Work out the finished part from the listing and answer in its coordinate system (mm). A direction names the side the tool comes from. Round coordinates to 2 decimals unless told otherwise and drop trailing zeros. Order: outer loops, then holes, each group sorted by start corner. A loop starts at its lowest first (then second) coordinate and runs counter-clockwise, first axis right, second up. Notation, with made-up numbers: M -7,-13.5 L 35,-13.5 A31 ccw 35,16.5 Z; hole C 86,85 d3. An arc over 180 degrees is marked long. Return JSON: item names as keys, results as strings.
from build123d import *

# Parameters (mm, degrees)
F0_W      = 205
F0_H      = 205
F0_W_2    = 195
F0_H_2    = 195
F1_DEPTH  = 200
F0_R      = 1.5
F0_W_3    = 55
F0_H_3    = 55
F2_DEPTH  = 3
F0_W_4    = 49
F0_H_4    = 49
F3_DEPTH  = 24
F4_W      = 46
F4_H      = 14
F5_DEPTH  = 60
F6_W      = 46
F6_H      = 14
F7_DEPTH  = 60
F8_W      = 49
F8_H      = 49
F9_DEPTH  = 4
F10_W     = 55
F10_H     = 55
F10_W_2   = 50
F10_H_2   = 50
F11_DEPTH = 150


with BuildPart() as f1:
    # F0 (on Top) → F1 (new body)
    with BuildSketch(Plane.XY):
        Rectangle(F0_W, F0_H)
        Rectangle(F0_W_2, F0_H_2, mode=Mode.SUBTRACT)
    extrude(amount=F1_DEPTH)

    # F0 (on Top) → F2 (join)
    with BuildSketch(Plane.XY):
        Rectangle(F0_W_2, F0_H_2)
        with Locations((-95.5, -95.5)):
            Circle(F0_R, mode=Mode.SUBTRACT)
        with Locations((-10, -48.9040691386)):
            Circle(F0_R, mode=Mode.SUBTRACT)
        with Locations((-48.9040691386, -10)):
            Circle(F0_R, mode=Mode.SUBTRACT)
        with Locations((95.5, -95.5)):
            Circle(F0_R, mode=Mode.SUBTRACT)
        with Locations((10, -48.9040691386)):
            Circle(F0_R, mode=Mode.SUBTRACT)
        with Locations((48.9040691386, -10)):
            Circle(F0_R, mode=Mode.SUBTRACT)
        with Locations((-48.9040691386, 10)):
            Circle(F0_R, mode=Mode.SUBTRACT)
        with Locations((-10, 48.9040691386)):
            Circle(F0_R, mode=Mode.SUBTRACT)
        with Locations((-95.5, 95.5)):
            Circle(F0_R, mode=Mode.SUBTRACT)
        Rectangle(F0_W_3, F0_H_3, mode=Mode.SUBTRACT)
        with Locations((48.9040691386, 10)):
            Circle(F0_R, mode=Mode.SUBTRACT)
        with Locations((10, 48.9040691386)):
            Circle(F0_R, mode=Mode.SUBTRACT)
        with Locations((95.5, 95.5)):
            Circle(F0_R, mode=Mode.SUBTRACT)
    extrude(amount=F2_DEPTH)

    # F0 (on Top) → F3 (join)
    with BuildSketch(Plane.XY):
        Rectangle(F0_W_3, F0_H_3)
        Rectangle(F0_W_4, F0_H_4, mode=Mode.SUBTRACT)
    extrude(amount=F3_DEPTH)

    # F4 (on face) → F5 (cut)
    with BuildSketch(Plane(origin=(-27.5, 0, 0), x_dir=(0, -1, 0), z_dir=(-1, 0, 0))):
        with Locations((0, 13.2578094924)):
            Rectangle(F4_W, F4_H)
    extrude(amount=-F5_DEPTH, mode=Mode.SUBTRACT)

    # F6 (on face) → F7 (cut)
    with BuildSketch(Plane(origin=(0, 27.5, 0), x_dir=(-1, 0, 0), z_dir=(0, 1, 0))):
        with Locations((0, 13.5)):
            Rectangle(F6_W, F6_H)
    extrude(amount=-F7_DEPTH, mode=Mode.SUBTRACT)

    # F8 (on face) → F9 (join)
    with BuildSketch(Plane.XY.offset(24)):
        Rectangle(F8_W, F8_H)
    extrude(amount=-F9_DEPTH)

    # F10 (on face) → F11 (join)
    with BuildSketch(Plane.XY.offset(24)):
        Rectangle(F10_W, F10_H)
        Rectangle(F10_W_2, F10_H_2, mode=Mode.SUBTRACT)
    extrude(amount=F11_DEPTH)


solid = f1.part
Item 1: Which of the six approach directions +Z, -Z, +X, -X, +Y, -Y give full straight-line access (tool end or side, diameter ignored) to faces 5 (the flat face through (-97.5, -1, 100)), 6 (the flat face through (-8, -98, 200)), 7 (the flat face through (0, 0, 20))?
Output:
{"face 5": "+Z", "face 6": "+Z, +X, -X, +Y, -Y", "face 7": "-Z"}
Item 2: Consider line 1 along X through (y, z) = (-27, 148.5); line 2 along X through (y, z) = (7.5, 121.5); line 3 along X through (y, z) = (86.5, 99). Determine where each line is inside the solid, lowest interval first. Write a range as [from, to].
Output:
{"line 1": "x = [-102.5, -97.5], [-27.5, 27.5], [97.5, 102.5]", "line 2": "x = [-102.5, -97.5], [-27.5, -25], [25, 27.5], [97.5, 102.5]", "line 3": "x = [-102.5, -97.5], [97.5, 102.5]"}
Item 3: Find section B-B (y = 70.5). Determine the outline of the cut face in (x, z).
Output:
{"outline": "M -102.5,0 L 102.5,0 L 102.5,200 L 97.5,200 L 97.5,3 L -97.5,3 L -97.5,200 L -102.5,200 Z"}
Item 4: Find section A-A (z = 35). Determine the outline of the cut face in (x, y).
Output:
{"outline": "M -102.5,-102.5 L 102.5,-102.5 L 102.5,102.5 L -102.5,102.5 Z; M -27.5,-27.5 L 27.5,-27.5 L 27.5,27.5 L -27.5,27.5 Z; hole M -97.5,-97.5 L 97.5,-97.5 L 97.5,97.5 L -97.5,97.5 Z; hole M -25,-25 L 25,-25 L 25,25 L -25,25 Z"}
Item 5: The mould has two halves that part along X. Classify faces 1 (the flat face through (-47, 1, 0)), 2 (the flat face through (0, 27.5, 87)), 3 (the flat face through (0, 25, 98)), 4 (the flat face through (-102.5, -1, 99)): pulls with the +X half, pulls with the -X half, needs draft (parallel to the pull), parting line crosses it, or undercut.
Output:
{"face 1": "needs draft", "face 2": "undercut", "face 3": "undercut", "face 4": "pulls with the -X half"}
Item 6: Each of these flat-tipped pins is pushed along its axis until it touches: pin 1 (5 mm diameter, centred on x = -47, y = 59.5, fed in from -Z); pin 2 (1.5 mm diameter, centred on x = 38.5, y = 41, fed in from +Z); pin 3 (24.5 mm diameter, centred on x = -5, y = -2, fed in from -Z); pin 4 (1.8 mm diameter, centred on x = -95.5, y = 95.5, fed in from +Z). Where does it stop, or does it pass through?
Output:
{"pin 1": "stops at z = 0", "pin 2": "stops at z = 3", "pin 3": "stops at z = 20", "pin 4": "passes through"}
Item 7: Find section C-C (z = 177). Determine the outline of the cut face in (x, y), plus the area to 3 significant figures.
Output:
{"outline": "M -102.5,-102.5 L 102.5,-102.5 L 102.5,102.5 L -102.5,102.5 Z; hole M -97.5,-97.5 L 97.5,-97.5 L 97.5,97.5 L -97.5,97.5 Z", "area": "4,000 mm^2"}
